from build123d import *

# Parameters (mm, degrees)
F0_R            = 2.54
F0_R_2          = 1.27
F1_DEPTH        = 1.6002
F3_DEPTH        = 1.6002
F3_COPIES_COUNT = 8
F5_R            = 0.254
F6_R            = 1.524
F7_DEPTH        = 0.508


# Not quite as in the source:
# - a pattern or mirror of a feature is missing from the dataset's text; its kind, count and spacing are read off the source's solid


with BuildPart() as f1:
    # F0 (on Front) → F1 (new body)
    with BuildSketch(Plane.XZ):
        Circle(F0_R)
        Circle(F0_R_2, mode=Mode.SUBTRACT)
    extrude(amount=F1_DEPTH)

    # F2 (on face) → F3 (join, through all)
    with BuildSketch(Plane.XZ.offset(1.6002)):
        Polygon((0.4233333333, 3.3866666667), (-0.4233333333, 3.3866666667), (-0.5926666667, 2.4698878967), (0.5926666667, 2.4698878967), align=None)
    f3 = extrude(amount=-F3_DEPTH)

    # F3_copies: F3 ×8 about axis
    f3_copies_axis = Axis((0, 0, 0), (0, 1, 0))
    for i in range(1, F3_COPIES_COUNT):
        add(f3.rotate(f3_copies_axis, i * 360 / F3_COPIES_COUNT))

    # F5
    f5_edges = [f1.edges().sort_by_distance(p)[0] for p in [
        (-0.423333, -0.8001, 3.386667),
        (-0.592667, -0.8001, 2.469888),
        (0.423333, -0.8001, 3.386667),
        (0.592667, -0.8001, 2.469888),
        (-1.327396, -0.8001, 2.165553),
        (-2.095393, -0.8001, 2.694077),
        (2.165553, -0.8001, 1.327396),
        (2.694077, -0.8001, 2.095393),
        (2.469888, -0.8001, 0.592667),
        (3.386667, -0.8001, 0.423333),
        (3.386667, -0.8001, -0.423333),
        (2.469888, -0.8001, -0.592667),
        (2.165553, -0.8001, -1.327396),
        (2.694077, -0.8001, -2.095393),
        (2.095393, -0.8001, -2.694077),
        (1.327396, -0.8001, -2.165553),
        (0.592667, -0.8001, -2.469888),
        (0.423333, -0.8001, -3.386667),
        (-0.423333, -0.8001, -3.386667),
        (-0.592667, -0.8001, -2.469888),
        (-1.327396, -0.8001, -2.165553),
        (-2.095393, -0.8001, -2.694077),
        (-2.694077, -0.8001, -2.095393),
        (-2.165553, -0.8001, -1.327396),
        (-2.469888, -0.8001, -0.592667),
        (-3.386667, -0.8001, -0.423333),
        (-3.386667, -0.8001, 0.423333),
        (-2.469888, -0.8001, 0.592667),
        (-2.165553, -0.8001, 1.327396),
        (1.327396, -0.8001, 2.165553),
        (2.095393, -0.8001, 2.694077),
        (-2.694077, -0.8001, 2.095393),
    ]]
    fillet(f5_edges, radius=F5_R)

    # F6 (on face) → F7 (cut)
    with BuildSketch(Plane(origin=(0, 0, 0), x_dir=(-1, 0, 0), z_dir=(0, 1, 0))):
        Circle(F6_R)
    extrude(amount=-F7_DEPTH, mode=Mode.SUBTRACT)


solid = f1.part
The listing builds one solid part. Answer for the finished solid, in the listing's coordinates (mm). Round coordinates to 2 decimals unless told otherwise and drop trailing zeros. Write each loop counter-clockwise with the first axis right and the second up, starting at its lowest first coordinate (ties: lowest second). Pieces come first, ordered by that corner, then holes. Notation, with made-up numbers: (-20, -38.5) - (24, -38.5) arc R19 cw to (24, -11.5) - close; hole circle Ø10 at (70, 87). An arc over 180 degrees is marked (long way). Use one line per item in the form item = value. Start each with the question number.
Item 1: Find the intervals of material crossed by line 1 (Z direction, x = 0, y = -0.4); line 2 (X direction, y = -0.9, z = 0), in increasing order. Write a range as [from, to].
Item 2: A cutting plane is placed at A-A (z = 0). Write down the section's boundary in (x, y), plus the area to 3 significant figures.
Item 3: A cutting plane is placed at B-B (x = 0). Write down the section's boundary in (y, z).
Item 4: Determine the mould class of faces 1 (the cylindrical face through (0.2, -0.25, 1.51)), 2 (the flat face through (-2, 0, 1)) for opening direction Z: +Z half, -Z half, draft (parallel to the pull), parting line (faces both ways), or undercut.
Item 5: A cutting plane is placed at C-C (x = 2.75). Write down the section's boundary in (y, z), plus the area to 3 significant figures.
The answers:
q1.line_1 = [-3.39, -1.52], [1.52, 3.39]
q1.line_2 = [-3.39, -1.27], [1.27, 3.39]
q2.outline = (-3.39, -1.6) - (-1.27, -1.6) - (-1.27, -0.51) - (-1.52, -0.51) - (-1.52, 0) - (-3.39, 0) - close; (1.27, -1.6) - (3.39, -1.6) - (3.39, 0) - (1.52, 0) - (1.52, -0.51) - (1.27, -0.51) - close
q2.area = 6.52 mm^2
q3.outline = (-1.6, -3.39) - (0, -3.39) - (0, -1.52) - (-0.51, -1.52) - (-0.51, -1.27) - (-1.6, -1.27) - close; (-1.6, 1.27) - (-0.51, 1.27) - (-0.51, 1.52) - (0, 1.52) - (0, 3.39) - (-1.6, 3.39) - close
q4.face_1 = undercut
q4.face_2 = draft
q5.outline = (-1.6, -0.54) - (0, -0.54) - (0, 0.54) - (-1.6, 0.54) - close
q5.area = 1.73 mm^2
